```python
from build123d import *

# Parameters (mm, degrees)
EXTRUDE_1_DEPTH     = 8
SKETCH_2_R          = 1.6
CUT_EXTRUDE_1_DEPTH = 8


with BuildPart() as part:
    # ｽｹｯﾁ1 → ﾎﾞｽ - 押し出し1 (new body)
    with BuildSketch(Plane.XY):
        with BuildLine():
            Line((-17.85, 0), (-20.85, 0))
            Line((-20.85, 0), (-20.85, -17.85))
            Line((-20.85, -17.85), (-29, -17.85))
            Line((-29, -17.85), (-29, -22.85))
            Line((-29, -22.85), (29, -22.85))
            Line((29, -22.85), (29, -17.85))
            Line((29, -17.85), (20.85, -17.85))
            Line((20.85, -17.85), (20.85, 0))
            Line((20.85, 0), (17.85, 0))
            ThreePointArc((17.85, 0), (0, -17.85), (-17.85, 0))
        make_face()
    extrude(amount=EXTRUDE_1_DEPTH)

    # ｽｹｯﾁ2 → ｶｯﾄ - 押し出し1 (cut)
    with BuildSketch(Plane.XZ.offset(22.85)):
        with Locations(Location((-25, 4, 0), (0, 0, 270))):
            Circle(SKETCH_2_R)
        with Locations(Location((25, 4, 0), (0, 0, 270))):
            Circle(SKETCH_2_R)
    extrude(amount=-CUT_EXTRUDE_1_DEPTH, mode=Mode.SUBTRACT)


solid = part.part
```
Check sheet for the modelled part. Datum: model origin and axes. Units: mm. A direction names the side the tool comes from. Round coordinates to 2 decimals unless told otherwise and drop trailing zeros. Write each loop counter-clockwise with the first axis right and the second up, starting at its lowest first coordinate (ties: lowest second). Pieces come first, ordered by that corner, then holes. Notation, with made-up numbers: M 8,37 L 32,37 A13 cw 32,61 Z; hole C 65.5,42 d4. An arc over 180 degrees is marked long. Write item = value, one per line. Start each with the question number.
1. Section check D-D, the plane z = 1.5. Record the cut outline in (x, y), then the cut area to 3 significant figures.
2. Scan lines: line 1 (X direction, y = -20.55, z = 4); line 2 (X direction, y = -13.75, z = 1); line 3 (X direction, y = -2.25, z = 4.75). Record each from-to range of solid material in increasing order. Write a range as [from, to].
3. Tool access check on faces 1 (the flat face through (25, -17.85, 6)), 2 (the flat face through (0, -19, 8)), 3 (the flat face through (-20.85, -9, 4)). Record the directions out of +Z, -Z, +X, -X, +Y, -Y that give a thin tool (end or side, any length) a straight path to the whole face; none if there is none.
4. Gauge pin test, flat ends, axial feed: pin 1 (1.5 mm diameter, centred on x = 12.5, z = 1.5, fed in from +Y); pin 2 (4 mm diameter, centred on x = -25, z = 4, fed in from +Y); pin 3 (3 mm diameter, centred on x = 25, z = 4, fed in from -Y). Record the tip position at first contact, or that the pin passes through.
5. Release check for a two-part mould opening along X. For faces 4 (the flat face through (0, -19, 0)), 5 (the flat face through (20.85, -9, 4)), 6 (the cylindrical face through (-23.414, -20.385, 4.208)) record: pulls with the +X half, pulls with the -X half, needs draft (parallel to the pull), parting line crosses it, or undercut.
6. Section check C-C, the plane y = -10.5. Record the cut outline in (x, z).
7. Section check A-A, the plane x = 25. Record the cut outline in (y, z).
8. Section check B-B, the plane z = 4. Record the cut outline in (x, y).
Results found:
q1.outline = M -29,-22.85 L 29,-22.85 L 29,-17.85 L 20.85,-17.85 L 20.85,0 L 17.85,0 A17.85 cw -17.85,0 L -20.85,0 L -20.85,-17.85 L -29,-17.85 Z
q1.area = 534 mm^2
q2.line_1 = [-29, -26.6], [-23.4, 23.4], [26.6, 29]
q2.line_2 = [-20.85, -11.38], [11.38, 20.85]
q2.line_3 = [-20.85, -17.71], [17.71, 20.85]
q3.face_1 = +Z, -Z, +X, +Y
q3.face_2 = +Z, +X, -X, +Y, -Y
q3.face_3 = +Z, -Z, -X, +Y
q4.pin_1 = -11.96
q4.pin_2 = -17.85
q4.pin_3 = through
q5.face_4 = needs draft
q5.face_5 = pulls with the +X half
q5.face_6 = undercut
q6.outline = M -20.85,0 L -14.44,0 L -14.44,8 L -20.85,8 Z; M 14.44,0 L 20.85,0 L 20.85,8 L 14.44,8 Z
q7.outline = M -22.85,0 L -17.85,0 L -17.85,2.4 L -22.85,2.4 Z; M -22.85,5.6 L -17.85,5.6 L -17.85,8 L -22.85,8 Z
q8.outline = M -29,-22.85 L -26.6,-22.85 L -26.6,-17.85 L -29,-17.85 Z; M -23.4,-22.85 L 23.4,-22.85 L 23.4,-17.85 L 20.85,-17.85 L 20.85,0 L 17.85,0 A17.85 cw -17.85,0 L -20.85,0 L -20.85,-17.85 L -23.4,-17.85 Z; M 26.6,-22.85 L 29,-22.85 L 29,-17.85 L 26.6,-17.85 Z
